Geometry: final body of the model. Coordinates: model frame, mm. Face numbers are marked on the shaded views. A direction names the side the tool comes from. Give positions to 0.01 mm unless a question says otherwise; leave off trailing zeros. Write each loop counter-clockwise with the first axis right and the second up, starting at its lowest first coordinate (ties: lowest second). Pieces come first, ordered by that corner, then holes.
Q1. Section A-A (z = 0). Return the cut outline in (x, y).
Q2. Line query: line 1 (Z direction, x = 0, y = 1.4); line 2 (X direction, y = 3, z = 0); line 3 (Z direction, x = -22, y = 2.25). Output: solid intervals per line, ascending.
Q3. Reachability of the marked faces 4 and 5 from +Z, -Z, +X, -X, +Y, -Y: full face, straight path, thin tool, end or side. Return the list, or none.
Q4. Section C-C (z = -40). Return the cut outline in (x, y).
Q5. Mould query, pull axis X, two halves, no side actions, for the marked faces 1, 2 and 3. Classes: +X half, -X half, draft (parallel to the pull), parting line (faces both ways), or undercut.
Q6. Pin query (flat end, axial travel): pin 1 Ø6 at (x, y) = (34, 7.5) entering from +Z; pin 2 Ø1.5 at (x, y) = (26, 3) entering from -Z. Return the tip coordinate at first contact, or that it passes through.
Q7. Section B-B (y = 7.5). State how many separate pieces and enclosed holes the cut face has, plus the area to 3 significant figures.
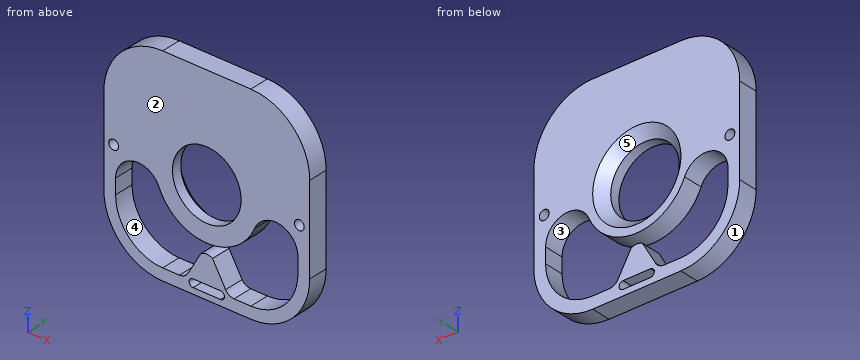
Autodesk Inventor part; units mm, degrees
ref_plane "YZ Plane" through (0, 0, 0) normal (1, 0, 0) x (0, 1, 0)
ref_plane "XZ Plane" through (0, 0, 0) normal (0, 1, 0) x (-1, 0, 0)
ref_plane "XY Plane" through (0, 0, 0) normal (0, 0, 1) x (1, 0, 0)
sketch "Sketch1" plane through (0, 0, 0) normal (0, 1, 0) x (-1, 0, 0)
  line L0 (52.5, 52.5) -> (-52.5, 52.5)
  line L1 (-52.5, 52.5) -> (-52.5, -52.5)
  line L2 (-52.5, -52.5) -> (52.5, -52.5)
  line L3 (52.5, -52.5) -> (52.5, 52.5)
  line L4 (52.5, 52.5) -> (-52.5, -52.5) construction
  line L5 (-52.5, 52.5) -> (52.5, -52.5) construction
  point P0 (0, 0)
  dimension "d0" = 105
  dimension "d1" = 105
extrude "Extrusion1" add sketch "Sketch1" along normal blind 10
fillet "Fillet1" radius 30 4 edges at (-52.5, 5, -52.5) (-52.5, 5, 52.5) (52.5, 5, -52.5) (52.5, 5, 52.5)
sketch "Sketch2" plane through (0, 10, 0) normal (0, 1, 0) x (1, 0, 0)
  circle A0 centre (0, 0) radius 17.5
  dimension "d5" = 35
extrude "Extrusion2" cut sketch "Sketch2" against normal blind 10
chamfer "Chamfer1" distance 5 angle 45 1 edges at (-17.5, 10, 0)
sketch "Sketch3" plane through (0, 10, 0) normal (0, 1, 0) x (1, 0, 0)
  arc A0 (22.5, -52.5) -> (52.5, -22.5) centre (22.5, -22.5) ccw
  line L0 (52.5, -22.5) -> (52.5, 22.5)
  arc A1 (52.5, 22.5) -> (22.5, 52.5) centre (22.5, 22.5) ccw
  line L1 (22.5, 52.5) -> (-22.5, 52.5)
  arc A2 (-22.5, 52.5) -> (-52.5, 22.5) centre (-22.5, 22.5) ccw
  line L2 (-52.5, 22.5) -> (-52.5, -22.5)
  arc A3 (-52.5, -22.5) -> (-22.5, -52.5) centre (-22.5, -22.5) ccw
  line L3 (-22.5, -52.5) -> (22.5, -52.5)
  circle A4 centre (0, 0) radius 22.5
  line L4 (46.5, 22.5) -> (46.5, -22.5)
  arc A5 (22.5, -46.5) -> (46.5, -22.5) centre (22.5, -22.5) ccw
  line L5 (22.5, -46.5) -> (-22.5, -46.5)
  arc A6 (-46.5, -22.5) -> (-22.5, -46.5) centre (-22.5, -22.5) ccw
  line L6 (-46.5, -22.5) -> (-46.5, 22.5)
  arc A7 (-22.5, 46.5) -> (-46.5, 22.5) centre (-22.5, 22.5) ccw
  line L7 (-22.5, 46.5) -> (22.5, 46.5)
  arc A8 (46.5, 22.5) -> (22.5, 46.5) centre (22.5, 22.5) ccw
  circle A9 centre (0, 0) radius 26.5
  arc A10 (24.4079, 10.3201) -> (46.5, 14.7986) centre (35, 14.7986) ccw
  arc A11 (-46.5, 14.7986) -> (-24.4079, 10.3201) centre (-35, 14.7986) ccw
  dimension "d11" = 6
  dimension "d12" = 4
  dimension "d13" = 23
  dimension "d14" = 23
extrude "Extrusion3" cut sketch "Sketch3" against normal blind 10 contours L4 A10 A9 A11 L6 A7 L7 A8
sketch "Sketch5" plane through (0, 10, 0) normal (0, 1, 0) x (1, 0, 0)
  line L0 (52.2088, 0) -> (47.2088, 0)
  line L1 (-52.5, 22.5) -> (-52.5, -22.5)
  line L2 (-52.5, 0) -> (-47.5, 0)
  circle A0 centre (47.2088, 0) radius 2.5
  circle A1 centre (-47.5, 0) radius 2.5
  point P0 (0, 0)
  dimension "d21" = 5
  dimension "d22" = 5
  dimension "d23" = 5
  dimension "d24" = 5
extrude "Extrusion4" cut sketch "Sketch5" against normal blind 10
sketch "Sketch6" plane through (0, 10, 0) normal (0, 1, 0) x (1, 0, 0)
  line L0 (52.5, 52.5) -> (14.5, 52.5)
  line L1 (22.5, 52.5) -> (-22.5, 52.5)
  line L2 (-52.5, 52.5) -> (-14.5, 52.5)
  line L3 (0, 52.5) -> (0, 31.5)
  line L4 (0, 31.5) -> (0, 37)
  arc A0 (-5.4968, 36.8121) -> (5.4968, 36.8121) centre (0, 37) ccw
  line L5 (14.5, 52.5) -> (2.9353, 32.3488)
  line L6 (-2.9353, 32.3488) -> (-14.5, 52.5)
  point P0 (0, 0)
  dimension "d27" = 38
  dimension "d28" = 38
  dimension "d29" = 21
  dimension "d30" = 5.5
  dimension "d31" = 11
extrude "Extrusion5" add sketch "Sketch6" against normal blind 10 contours L5 A0 L3 L1 | L3 A0 L6 L1
fillet "Fillet2" radius 5 2 edges at (11.0566, 5, -46.5) (-11.0566, 5, -46.5)
sketch "Sketch7" plane through (0, 10, 0) normal (0, 1, 0) x (1, 0, 0)
  line L0 (22.5, 52.5) -> (-22.5, 52.5)
  line L1 (0, 47.5) -> (-7, 47.5)
  line L2 (-7, 47.5) -> (7, 47.5)
  arc A0 (7, 45.5) -> (7, 49.5) centre (7, 47.5) ccw
  arc A1 (-7, 49.5) -> (-7, 45.5) centre (-7, 47.5) ccw
  line L3 (7, 45.5) -> (-7, 45.5)
  line L4 (-7, 49.5) -> (7, 49.5)
  point P0 (0, 0)
  dimension "d37" = 14
  dimension "d38" = 4
  dimension "d39" = 4
extrude "Extrusion6" cut sketch "Sketch7" against normal blind 10
properties part number "Del 6"
Computed:
1. outline: (-52.5, 0) - (-50, 0) - (-50, 10) - (-52.5, 10) - close; (-45, 0) - (-17.5, 0) - (-17.5, 5) - (-22.5, 10) - (-45, 10) - close; (17.5, 0) - (44.71, 0) - (44.71, 10) - (22.5, 10) - (17.5, 5) - close; (49.71, 0) - (52.5, 0) - (52.5, 10) - (49.71, 10) - close
2. line 1: z = -52.5 to -49.5, -45.5 to -31.5, -26.5 to -17.5, 17.5 to 52.5
2. line 2: x = -52.5 to -50, -45 to -17.5, 17.5 to 44.71, 49.71 to 52.5
2. line 3: z = -52.5 to -46.5, -14.77 to 52.5
3. face 4: +Y, -Y
3. face 5: +Y
4. outline: (-46.87, 0) - (-38.92, 0) - (-38.92, 10) - (-46.87, 10) - close; (-7.33, 0) - (7.33, 0) - (7.33, 10) - (-7.33, 10) - close; (38.92, 0) - (46.87, 0) - (46.87, 10) - (38.92, 10) - close
5. face 1: -X half
5. face 2: draft
5. face 3: undercut
6. pin 1: stops at z = 51.27
6. pin 2: stops at z = -52.37
7. separate pieces: 1
7. enclosed holes: 5
7. area: 6,330 mm2
